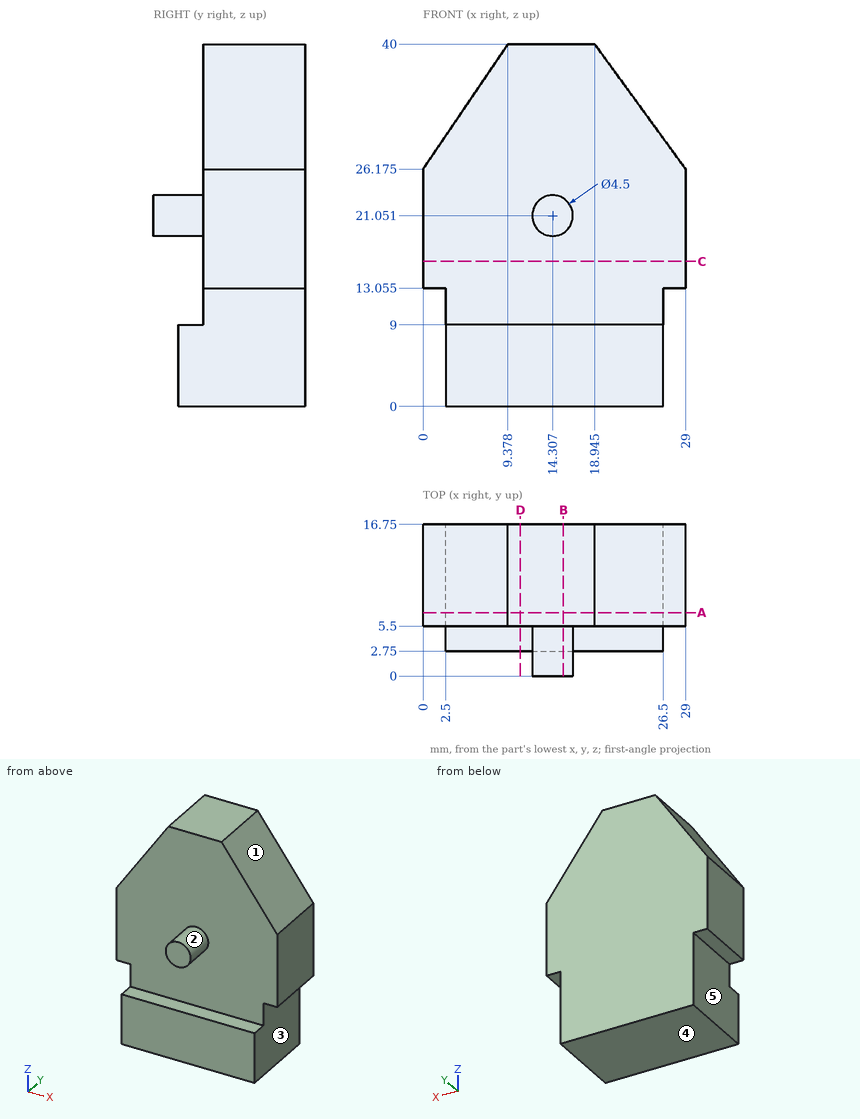
Verification items for this drawing (mm, ordinates from the low corner). A direction names the side the tool comes from. Coordinates: 2 decimals unless noted, no trailing zeros. Write each loop counter-clockwise with the first axis right and the second up, starting at its lowest first coordinate (ties: lowest second). Pieces come first, ordered by that corner, then holes. Notation, with made-up numbers: (34, 51.25) - (51, 51.25) arc R17 cw to (51, 61.25) - close; hole circle Ø7 at (57, 14.5). An arc over 180 degrees is marked (long way). One line per question, with ' | ' between items.
Item 1: Sectioned sample at B-B on x = 15.5. Record the boundary of the cut face in (y, z), plus the area to 3 significant figures.
Determined:
outline: (0, 19.14) - (5.5, 19.14) - (5.5, 9) - (2.75, 9) - (2.75, 0) - (16.75, 0) - (16.75, 40) - (5.5, 40) - (5.5, 22.96) - (0, 22.96) - close | area: 496 mm2
Item 2: Sectioned sample at C-C on z = 16. Record the boundary of the cut face in (x, y).
Determined:
outline: (0, 5.5) - (29, 5.5) - (29, 16.75) - (0, 16.75) - close
Item 3: Gauge pin test, flat ends, axial feed: P1, Ø10, axis at x = 8.5, z = 3.5, coming from the -Y side; P2, Ø0.8, axis at x = 1.5, y = 11, coming from the -Z side (1 decimal). Record the tip position at first contact, or that the pin passes through.
Determined:
P1: stops at y = 2.75 | P2: stops at z = 13.1
Item 4: Sectioned sample at D-D on x = 10.75. Record the boundary of the cut face in (y, z).
Determined:
outline: (2.75, 0) - (16.75, 0) - (16.75, 40) - (5.5, 40) - (5.5, 9) - (2.75, 9) - close
Item 5: Mould release check, pull along Z, two halves, no side actions. Record for the marked faces 1, 2 and 3: pulls with the +Z half, pulls with the -Z half, needs draft (parallel to the pull), parting line crosses it, or undercut.
Determined:
face 1: pulls with the +Z half | face 2: undercut | face 3: needs draft
Item 6: Thickness scan on line 1 (Y direction, x = 19.75, z = 4); line 2 (Y direction, x = 11.75, z = 20); line 3 (X direction, y = 16.25, z = 8). Record the ranges inside material, lowest first. Write a range as [from, to].
Determined:
line 1: y = [2.75, 16.75] | line 2: y = [5.5, 16.75] | line 3: x = [2.5, 26.5]
Item 7: Sectioned sample at A-A on y = 7. Record the boundary of the cut face in (x, z) (1 decimal), plus the area to 3 significant figures.
Determined:
outline: (0, 13.1) - (2.5, 13.1) - (2.5, 0) - (26.5, 0) - (26.5, 13.1) - (29, 13.1) - (29, 26.2) - (18.9, 40) - (9.4, 40) - (0, 26.2) - close | area: 960 mm2
Item 8: Access from +Z, -Z, +X, -X, +Y, -Y to the whole of each face (thin tool, end or side, straight path). Record for the marked faces 4 and 5.
Determined:
face 4: -Z, +X, -X, +Y, -Y | face 5: -Z, -X, +Y, -Y
